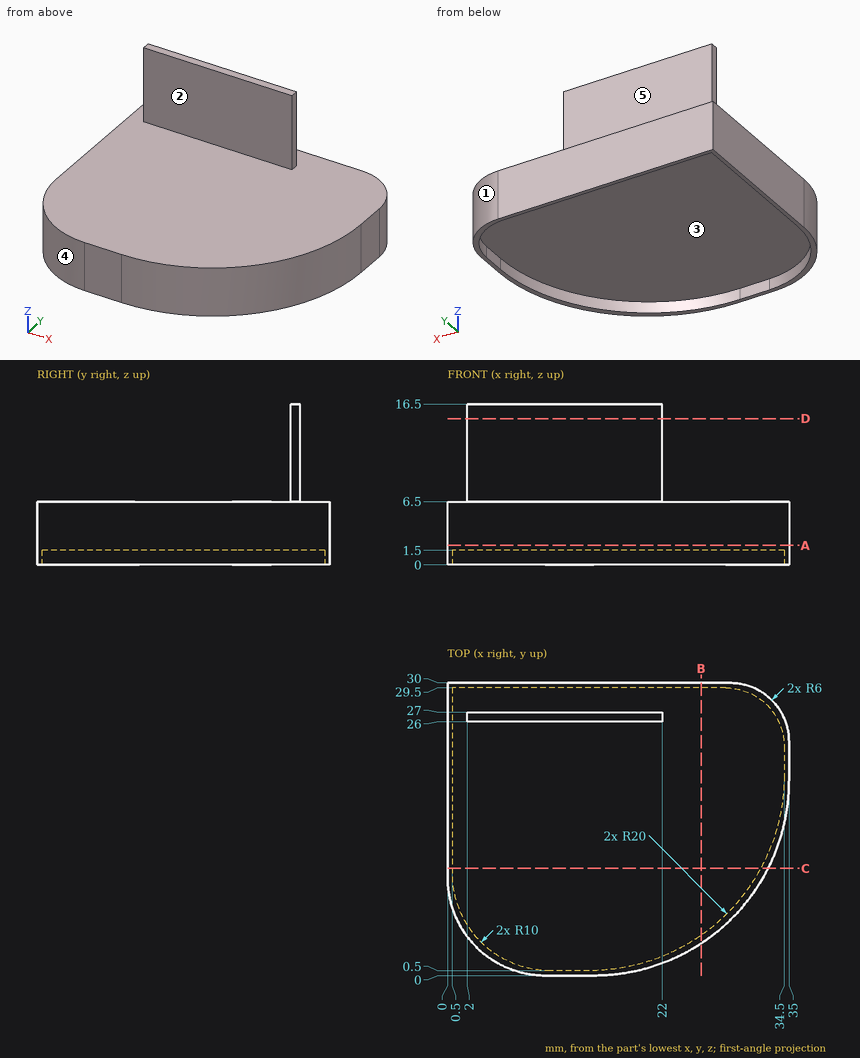
Could you check a few things on this drawing? It's one solid part, dimensions in mm from its lowest x, y, z. A direction names the side the tool comes from. Give positions to 0.01 mm unless a question says otherwise; leave off trailing zeros. Order: outer loops, then holes, each group sorted by start corner. A loop starts at its lowest first (then second) coordinate and runs counter-clockwise, first axis right, second up. Notation, with made-up numbers: (-19, -17) - (34, -17) arc R17 ccw to (34, -8) - close; hole circle Ø4 at (-35.5, 79.25). An arc over 180 degrees is marked (long way). Answer as a JSON object with one key per item and string values. Group by question number.
Item 1: For P1, Ø1, axis at x = 5, y = 9.5, coming from the -Z side; P2, Ø2, axis at x = 19, z = 14, coming from the +Y side; P3, Ø9, axis at x = 12.5, y = 8.5, coming from the +Z side, each with a flat end and sliding along its axis, tell me the tip position at first contact or that it passes through.
Item 2: If we section it at A-A on z = 2: Please give me the cut outline in (x, y), and give its area (3 significant figures).
Item 3: If we section it at C-C on y = 11: Please give me the cut outline in (x, z), and give its area (3 significant figures).
Item 4: If we section it at B-B on x = 26: Please give me the cut outline in (y, z).
Item 5: If we mould it in two halves opening along Y, with no side actions, what happens to the marked faces 1, 2 and 3? For each: pulls with the +Y half, pulls with the -Y half, needs draft (parallel to the pull), parting line crosses it, or undercut.
Item 6: Please list where these lines run through material, in increasing order: probe 1 along Z at (x, y) = (20.5, 7); probe 2 along Y at (x, z) = (12.5, 12); probe 3 along X at (y, z) = (17, 2.25).
Item 7: If we section it at D-D on z = 15: Please give me the cut outline in (x, y), and give its area (3 significant figures).
Item 8: Which directions (+Z, -Z, +X, -X, +Y, -Y) give clear straight access to the entire face, cutting with the end or side of a thin tool? Please do the marked faces 4 and 5.
Result set:
{
 "1": {"P1": "z = 1.5", "P2": "y = 27", "P3": "z = 6.5"},
 "2": {"outline": "(0, 10) arc R10 ccw to (10, 0) - (15, 0) arc R20 ccw to (35, 20) - (35, 24) arc R6 ccw to (29, 30) - (0, 30) - close", "area": "935 mm²"},
 "3": {"outline": "(0, 0) - (0.5, 0) - (0.5, 1.5) - (32.1, 1.5) - (32.1, 0) - (32.86, 0) - (32.86, 6.5) - (0, 6.5) - close", "area": "166 mm²"},
 "4": {"outline": "(3.3, 0) - (4.14, 0) - (4.14, 1.5) - (29.5, 1.5) - (29.5, 0) - (30, 0) - (30, 6.5) - (3.3, 6.5) - close"},
 "5": {"face 1": "pulls with the +Y half", "face 2": "pulls with the -Y half", "face 3": "undercut"},
 "6": {"probe 1": "1.5 to 6.5", "probe 2": "26 to 27", "probe 3": "0 to 34.77"},
 "7": {"outline": "(2, 26) - (22, 26) - (22, 27) - (2, 27) - close", "area": "20.0 mm²"},
 "8": {"face 4": "+Z, -Z, -X, -Y", "face 5": "+Z, +X, -X, +Y"}
}
